Geometry: final body of the model. Coordinates: model frame, mm. Coordinates: 2 decimals unless noted, no trailing zeros. Loops run counter-clockwise (first coordinate to the right, second up) from the corner with the lowest first, then second, coordinate; pieces in that order, holes last. Notation, with made-up numbers: (35.5, -18) -> (57.5, -18) arc R22 ccw to (57.5, 4) -> close; hole circle Ø7 at (11.5, 32.25). An arc over 180 degrees is marked (long way). One line per item, written item: value. Start each with the question number.
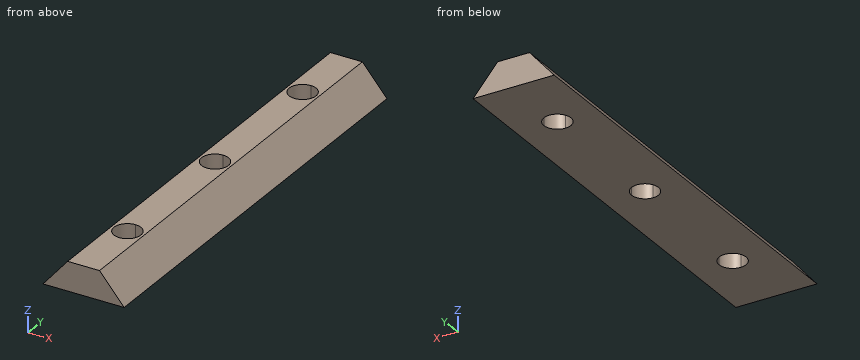
from build123d import *

# Parameters (mm, degrees)
F1_DEPTH = 75
F3_DEPTH = 5


with BuildPart() as f1:
    # F0 (on Front) → F1 (new body)
    with BuildSketch(Plane.XZ):
        Polygon((4.25, 5), (0, 0), (7, 0), (7, 5), align=None)
        Polygon((7, 5), (7, 0), (14, 0), (9.75, 5), align=None)
    extrude(amount=F1_DEPTH)

    # F2 (on face) → F3 (cut, through all)
    with BuildSketch(Plane.XY.offset(5)):
        with BuildLine():
            ThreePointArc((7, -14.825), (8.644023, -14.144023), (9.325, -12.5))
            ThreePointArc((9.325, -12.5), (8.644023, -10.855977), (7, -10.175))
            Line((7, -10.175), (7, -14.825))
        make_face()
        with BuildLine():
            ThreePointArc((9.325, -62.5), (8.644023, -60.855977), (7, -60.175))
            Line((7, -60.175), (7, -64.825))
            ThreePointArc((7, -64.825), (8.644023, -64.144023), (9.325, -62.5))
        make_face()
        with BuildLine():
            Line((7, -64.825), (7, -60.175))
            ThreePointArc((7, -60.175), (4.675, -62.5), (7, -64.825))
        make_face()
        with BuildLine():
            ThreePointArc((9.325, -37.5), (8.644023, -35.855977), (7, -35.175))
            Line((7, -35.175), (7, -39.825))
            ThreePointArc((7, -39.825), (8.644023, -39.144023), (9.325, -37.5))
        make_face()
        with BuildLine():
            Line((7, -39.825), (7, -35.175))
            ThreePointArc((7, -35.175), (4.675, -37.5), (7, -39.825))
        make_face()
        with BuildLine():
            Line((7, -14.825), (7, -10.175))
            ThreePointArc((7, -10.175), (4.675, -12.5), (7, -14.825))
        make_face()
    extrude(amount=-F3_DEPTH, mode=Mode.SUBTRACT)


solid = f1.part
1. Section D-D on x = 3. Return the cut outline in (y, z), plus the area to 3 significant figures.
2. Section C-C on y = -50. Return the cut outline in (x, z).
3. Section B-B on y = -64. Return the cut outline in (x, z), plus the area to 3 significant figures.
4. Line query: L1, parallel to Y at x = 5.75, z = 2.2; L2, parallel to Y at x = 6.25, z = 1.85; L3, parallel to X at y = -12, z = 1.8. Output: solid intervals per line, ascending. Write a range as [from, to].
5. Pin query (flat end, axial travel): pin 1 Ø2 at (y, z) = (-59.5, 2) entering from +X; pin 2 Ø2 at (y, z) = (-19, 1.5) entering from +X (3 decimals). Return the tip coordinate at first contact, or that it passes through.
6. Section A-A on z = 3.2. Return the cut outline in (x, y) (3 decimals).
Checks:
1. outline: (-75, 0) -> (0, 0) -> (0, 3.53) -> (-75, 3.53) -> close
1. area: 265 mm²
2. outline: (0, 0) -> (14, 0) -> (9.75, 5) -> (4.25, 5) -> close
3. outline: (0, 0) -> (5.22, 0) -> (5.22, 5) -> (4.25, 5) -> close; (8.78, 0) -> (14, 0) -> (9.75, 5) -> (8.78, 5) -> close
3. area: 31.0 mm²
4. L1: [-75, -64.46], [-60.54, -39.46], [-35.54, -14.46], [-10.54, 0]
4. L2: [-75, -64.7], [-60.3, -39.7], [-35.3, -14.7], [-10.3, 0]
4. L3: [1.53, 4.73], [9.27, 12.47]
5. pin 1: x = 13.15
5. pin 2: x = 13.575
6. outline: (2.72, -75) -> (11.28, -75) -> (11.28, 0) -> (2.72, 0) -> close; hole (7, -60.175) arc R2.325 ccw (long way) to (9.325, -62.5) arc R2.325 ccw to start; hole (7, -35.175) arc R2.325 ccw (long way) to (9.325, -37.5) arc R2.325 ccw to start; hole (7, -10.175) arc R2.325 ccw (long way) to (9.325, -12.5) arc R2.325 ccw to start
